Source: CAD feature listing. Evaluate the final solid. Frame: model axes, mm. A direction names the side the tool comes from. Coordinates: 2 decimals unless noted, no trailing zeros. Order: outer loops, then holes, each group sorted by start corner. A loop starts at its lowest first (then second) coordinate and runs counter-clockwise, first axis right, second up. Notation, with made-up numbers: (37, -37.5) -> (77, -37.5) arc R9 ccw to (77, -32.5) -> close; hole circle Ø4 at (10, 28.5). An arc over 180 degrees is marked (long way). Put each result on its own line as item: value.
from build123d import *

# Parameters (mm, degrees)
BOSS_EXTRUDE2_DEPTH = 3


with BuildPart() as part:
    # Sketch4 → Boss-Extrude2 (new body)
    with BuildSketch(Plane(origin=(0, 0, 0), x_dir=(1, 0, 0), z_dir=(0, 1, 0))):
        Polygon((-26, -90), (-9.5, -90), (-9.5, -87), (15.5, -87), (15.5, -90), (32, -90), (32, -78), (29, -78), (29, -56), (32, -56), (32, -34), (29, -34), (29, -12), (32, -12), (32, 0), (15.5, 0), (15.5, -3), (-9.5, -3), (-9.5, 0), (-26, 0), (-26, -12), (-23, -12), (-23, -34), (-26, -34), (-26, -56), (-23, -56), (-23, -78), (-26, -78), align=None)
        with BuildLine():
            Line((-20.2, -47.197183378), (-20.2, -5.849521076))
            ThreePointArc((-20.2, -5.849521076), (26.637033052, -34.647238196), (0.473831151, -83.005309319))
            Line((0.473831151, -83.005309319), (-20.2, -47.197183378))
        make_face(mode=Mode.SUBTRACT)
    extrude(amount=BOSS_EXTRUDE2_DEPTH)


solid = part.part
1. Cut plane B-B on z = 45. Output: boundary loops of the cut face in (x, y), plus the area to 3 significant figures.
Numbers:
outline: (-26, 0) -> (-20.2, 0) -> (-20.2, 3) -> (-26, 3) -> close; (28, 0) -> (32, 0) -> (32, 3) -> (28, 3) -> close
area: 29.4 mm2
2. Cut plane A-A on x = 12. Output: boundary loops of the cut face in (y, z).
Numbers:
outline: (0, 3) -> (3, 3) -> (3, 13) -> (0, 13) -> close; (0, 77) -> (3, 77) -> (3, 87) -> (0, 87) -> close
3. Pull-direction query (Z, two-part tool) for faces 6 (the flat face through (30, 1, 56)), 7 (the flat face through (-9.5, 1, 89)), 8 (the flat face through (3, 1, 87)); classes: pulls with the +Z half, pulls with the -Z half, needs draft (parallel to the pull), parting line crosses it, or undercut.
Numbers:
face 6: undercut
face 7: needs draft
face 8: pulls with the +Z half
4. First-contact query: pin 1 (0.9 mm diameter, centred on y = 1.5, z = 27, fed in from +X); pin 2 (3 mm diameter, centred on x = -13.5, z = 54, fed in from -Y); pin 3 (1 mm diameter, centred on y = 0.5, z = 64, fed in from -X); pin 4 (1.5 mm diameter, centred on x = 9, y = 2, fed in from +Z). Flat tips, straight axial feed; report the tip coordinate or a pass-through.
Numbers:
pin 1: stops at x = 29
pin 2: passes through
pin 3: stops at x = -23
pin 4: stops at z = 87
5. Ray query, line 1 along X through (y, z) = (1.5, 13.5); line 2 along X through (y, z) = (0.55, 55); line 3 along Z through (x, y) = (17.5, 1.3). Return the intervals inside material, ascending.
Numbers:
line 1: x = -23 to -20.2, 12.65 to 29
line 2: x = -26 to -15.7, 26.73 to 32
line 3: z = 0 to 17.99, 72.01 to 90
6. Set-up query: faces 1 (the flat face through (3, 1, 3)), 2 (the flat face through (-24, 1, 78)), 3 (the flat face through (-20.2, 1, 27)), 4 (the flat face through (29, 1, 23)), 5 (the flat face through (15.5, 1, 88)). Return all of +Z, -Z, +X, -X, +Y, -Y with unobstructed straight access to the full face (end or side cutting, diameter ignored); none if empty.
Numbers:
face 1: -Z, +Y, -Y
face 2: -X, +Y, -Y
face 3: +Y, -Y
face 4: +X, +Y, -Y
face 5: +Z, +Y, -Y
